Check sheet for the drawn part. Datum: minimum x, y, z corner. Units: mm. A direction names the side the tool comes from. Coordinates: 2 decimals unless noted, no trailing zeros. Loops run counter-clockwise (first coordinate to the right, second up) from the corner with the lowest first, then second, coordinate; pieces in that order, holes last. Notation, with made-up numbers: (52.5, 71.5) -> (74.5, 71.5) arc R21 ccw to (74.5, 75.5) -> close; hole circle Ø7 at (-24.75, 39.25). An arc over 180 degrees is marked (long way). Use CSV: the item, a comma, the result in double quotes. Start each with the question number.
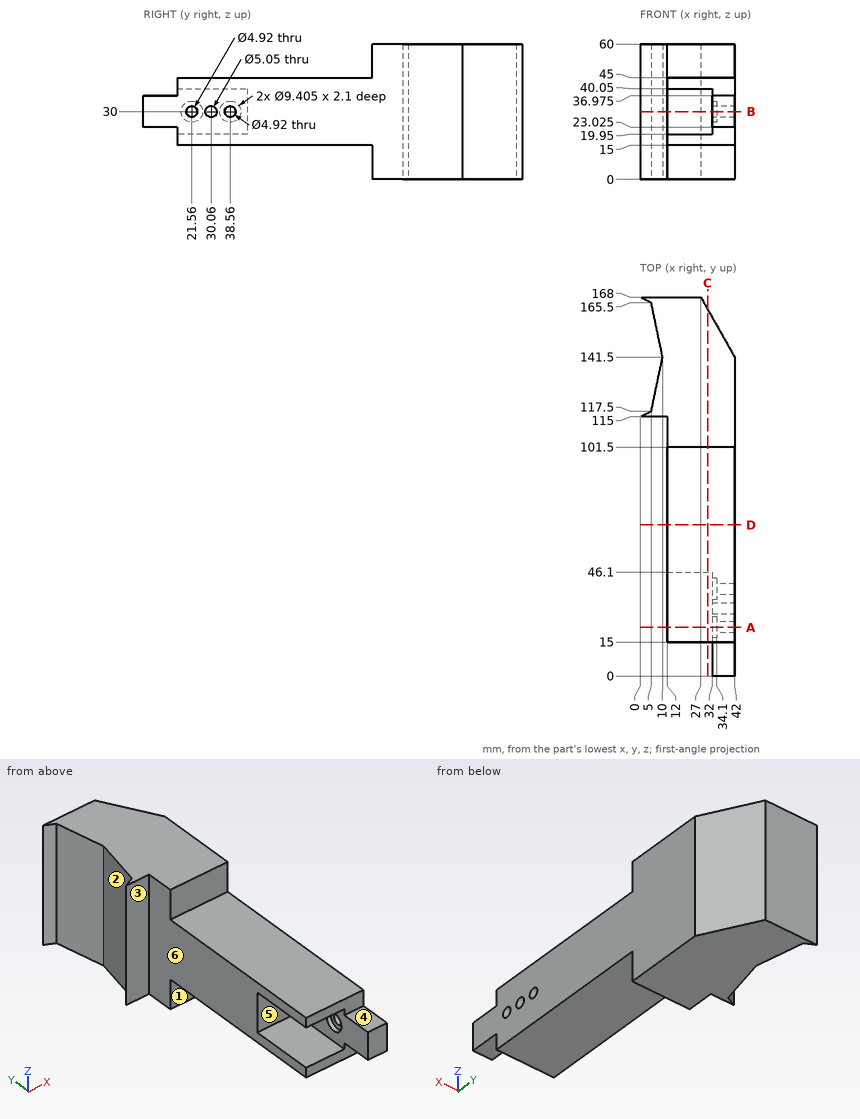
1. Release check for a two-part mould opening along Z. For the marked faces 4, 5 and 6 record: released by +Z, released by -Z, zero draft, split by the parting line, or undercut.
2. Scan lines: line 1 (Z direction, x = 36.5, y = 21.56); line 2 (Y direction, x = 33, z = 30) (1 decimal); line 3 (Y direction, x = 33.6, z = 30) (1 decimal). Record each from-to range of solid material in increasing order.
3. Cross-section at B-B, the plane z = 30. State how many separate pieces and enclosed holes the cut face has, plus the area to 3 significant figures.
4. Cross-section at A-A, the plane y = 21.56. Record the boundary of the cut face in (x, z), plus the area to 3 significant figures.
5. Depth check by flat-ended pin: pin 1 (10.5 mm diameter, centred on y = 19.5, z = 30.5, fed in from -X); pin 2 (22 mm diameter, centred on y = 33.5, z = 28.5, fed in from -X); pin 3 (2.5 mm diameter, centred on x = 34.5, z = 40, fed in from -Y); pin 4 (3 mm diameter, centred on x = 7, y = 144.5, fed in from -Z). Enter the tip coordinate at first touch or a pass-through.
6. Set-up check for the marked faces 1, 2 and 3: record each of +Z, -Z, +X, -X, +Y, -Y from which the full face is reachable in a straight line by a thin tool's end or side.
7. Cross-section at D-D, the plane y = 67. Record the boundary of the cut face in (x, z).
8. Cross-section at C-C, the plane x = 30. Record the boundary of the cut face in (y, z), plus the area to 3 significant figures.
Solution:
1,face 4,"released by +Z"
1,face 5,"undercut"
1,face 6,"zero draft"
2,line 1,"z = 15 to 27.54, 32.46 to 45"
2,line 2,"y = 0 to 16.9, 26.3 to 27.5, 32.6 to 33.9, 43.3 to 157.4"
2,line 3,"y = 0 to 16.9, 26.3 to 27.5, 32.6 to 33.9, 43.3 to 156.3"
3,separate pieces,"4"
3,enclosed holes,"0"
3,area,"4,020 mm2"
4,outline,"(12, 15) -> (42, 15) -> (42, 27.54) -> (34.1, 27.54) -> (34.1, 25.3) -> (32, 25.3) -> (32, 19.95) -> (12, 19.95) -> close; (12, 40.05) -> (32, 40.05) -> (32, 34.7) -> (34.1, 34.7) -> (34.1, 32.46) -> (42, 32.46) -> (42, 45) -> (12, 45) -> close"
4,area,"439 mm2"
5,pin 1,"stops at x = 32"
5,pin 2,"stops at x = 12"
5,pin 3,"stops at y = 15"
5,pin 4,"passes through"
6,face 1,"-Z, +X, -X, -Y"
6,face 2,"+Z, -Z, -X"
6,face 3,"+Z, -Z, -X, -Y"
7,outline,"(12, 15) -> (42, 15) -> (42, 45) -> (12, 45) -> close"
8,outline,"(15, 15) -> (101.5, 15) -> (101.5, 0) -> (162.7, 0) -> (162.7, 60) -> (101.5, 60) -> (101.5, 45) -> (15, 45) -> (15, 40.05) -> (46.1, 40.05) -> (46.1, 19.95) -> (15, 19.95) -> close"
8,area,"5,640 mm2"
